Work out the finished part from the listing and answer in its coordinate system (mm). Face numbers are marked on the shaded views. A direction names the side the tool comes from. Give positions to 0.01 mm unless a question says otherwise; leave off trailing zeros. Order: outer loops, then holes, each group sorted by start corner. A loop starts at its lowest first (then second) coordinate and runs counter-clockwise, first axis right, second up. Notation, with made-up numbers: (32.5, -13.5) - (78.5, -13.5) arc R31 cw to (78.5, 21.5) - close; hole circle Ø7 at (-20, 68.25). An arc over 180 degrees is marked (long way). Put each result on its own line as item: value.
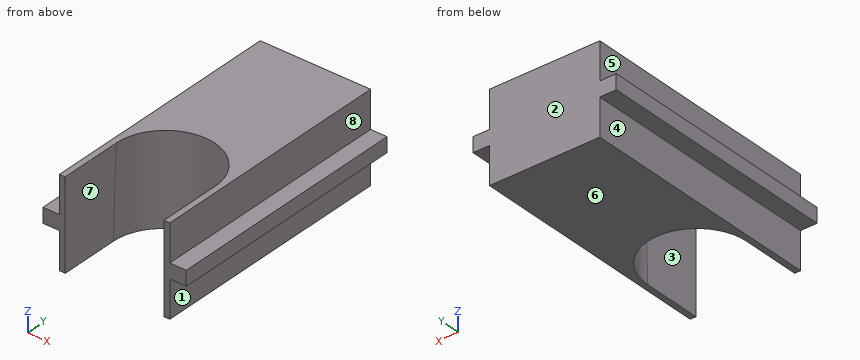
Autodesk Inventor part; units mm, degrees
ref_plane "YZ Plane" through (0, 0, 0) normal (1, 0, 0) x (0, 1, 0)
ref_plane "XZ Plane" through (0, 0, 0) normal (0, 1, 0) x (-1, 0, 0)
ref_plane "XY Plane" through (0, 0, 0) normal (0, 0, 1) x (1, 0, 0)
sketch "草圖1" plane through (0, 0, 0) normal (0, 1, 0) x (-1, 0, 0)
  line L0 (-33.5, 27) -> (33.5, 27)
  line L1 (33.5, 27) -> (33.5, -27)
  line L2 (33.5, -27) -> (-33.5, -27)
  line L3 (-33.5, -27) -> (-33.5, 27)
  line L4 (-33.5, 27) -> (33.5, -27) construction
  line L5 (33.5, 27) -> (-33.5, -27) construction
  line L6 (43.5, -4.5) -> (33.5, -4.5)
  line L7 (33.5, -4.5) -> (33.5, 4.5)
  line L8 (33.5, 4.5) -> (43.5, 4.5)
  line L9 (43.5, 4.5) -> (43.5, -4.5)
  line L10 (-33.5, -4.5) -> (-43.5, -4.5)
  line L11 (-43.5, -4.5) -> (-43.5, 4.5)
  line L12 (-43.5, 4.5) -> (-33.5, 4.5)
  line L13 (-33.5, 4.5) -> (-33.5, -4.5)
  point P0 (0, 0)
  point P1 (33.5, 0)
  point P2 (-33.5, 0)
  point P3 (-33.5, 4.5)
  point P4 (-33.5, -4.5)
  dimension "d0" = 67
  dimension "d1" = 54
  dimension "d2" = 9
  dimension "d3" = 10
extrude "擠出1" add sketch "草圖1" along normal blind 200
sketch "草圖2" plane through (-33.5, 0, 27) normal (0, 0, 1) x (1, 0, 0)
  circle A0 centre (33.5, 78) radius 30
  line L0 (0, 0) -> (67, 0)
  line L1 (3.5, 78) -> (63.5, 78)
  line L2 (63.5, 78) -> (63.5, -10.8713)
  line L3 (63.5, -10.8713) -> (3.5, -10.8713)
  line L4 (3.5, -10.8713) -> (3.5, 78)
  point P0 (33.5, 0)
  point P1 (33.5, 0)
  point P2 (63.5, 78)
  dimension "d6" = 78
  dimension "d7" = 60
extrude "擠出2" cut sketch "草圖2" against normal through all
sketch "草圖3" plane through (-33.5, 200, 27) normal (0, 0, 1) x (1, 0, 0)
  line L0 (-51.5496, -150) -> (118.5496, -150)
  line L1 (118.5496, -150) -> (118.5496, -200)
  line L2 (118.5496, -200) -> (-51.5496, -200)
  line L3 (-51.5496, -200) -> (-51.5496, -150)
  point P0 (33.5, -200)
  point P1 (33.5, -200)
  dimension "d10" = 50
extrude "擠出3" cut sketch "草圖3" against normal through all
sketch "草圖4" plane through (33.5, 200, -27) normal (0, 0, -1) x (-1, 0, 0)
  arc A0 (63.5, -122) -> (3.5, -122) centre (33.5, -122) ccw construction
  circle A1 centre (33.5, -114) radius 30
  line L0 (63.5, -150) -> (3.5, -150)
  line L1 (3.5, -150) -> (3.5, -114)
  line L2 (3.5, -114) -> (63.5, -114)
  line L3 (63.5, -114) -> (63.5, -150)
  point P0 (33.5, -200)
  point P1 (63.5, -150)
  dimension "d13" = 8
  dimension "d14" = 60
sketch "草圖5" plane through (-33.5, 200, 27) normal (0, 0, 1) x (1, 0, 0)
  arc A0 (63.5, -122) -> (3.5, -122) centre (33.5, -122) ccw construction
  circle A1 centre (33.5, -112) radius 30
  line L0 (63.5, -150) -> (3.5, -150)
  line L1 (3.5, -150) -> (3.5, -112)
  line L2 (3.5, -112) -> (63.5, -112)
  line L3 (63.5, -112) -> (63.5, -150)
  point P0 (33.5, -200)
  point P1 (63.5, -150)
  dimension "d15" = 10
  dimension "d16" = 60
loft "斷面混成1" cut profiles "草圖4", "草圖5"
properties part number "Slider-3"
(1) Given pin 1 (3 mm diameter, centred on x = 22.5, z = -14.5, fed in from -Y); pin 2 (7 mm diameter, centred on y = 106, z = -17, fed in from -X); pin 3 (25 mm diameter, centred on y = 109.5, z = -18, fed in from +X); pin 4 (25 mm diameter, centred on y = 120, z = 11.5, fed in from -X), each flat-ended and moving along its own axis, determine where each tip first touches the part or whether it passes through.
Geometry check:
pin 1: stops at y = 104.46
pin 2: stops at x = -33.5
pin 3: stops at x = 33.5
pin 4: stops at x = -43.5
(2) Straight lines are drawn through the part: line 1 (X direction, y = 70.5, z = 12); line 2 (X direction, y = 96, z = -7); line 3 (Z direction, x = -39, y = 116.5). For each, find the intervals that lie inside material, in ascending order.
Geometry check:
line 1: x = -33.5 to -30, 30 to 33.5
line 2: x = -33.5 to -28.54, 28.54 to 33.5
line 3: z = -4.5 to 4.5
(3) Section A-A, the plane y = 168.5 is taken. Write down the section's boundary in (x, z).
Geometry check:
outline: (-43.5, -4.5) - (-33.5, -4.5) - (-33.5, -27) - (33.5, -27) - (33.5, -4.5) - (43.5, -4.5) - (43.5, 4.5) - (33.5, 4.5) - (33.5, 27) - (-33.5, 27) - (-33.5, 4.5) - (-43.5, 4.5) - close
(4) A tool of negligible diameter and unlimited length cuts with its end or side. For the marked faces 1, 2, 3, 4 and 5, from which of +Z, -Z, +X, -X, +Y, -Y can it reach the whole face along a straight path? Write none if from no direction.
Geometry check:
face 1: -Z, +X, +Y, -Y
face 2: +Z, -Z, +X, -X, +Y
face 3: +Z, -Z, -Y
face 4: -Z, -X, +Y, -Y
face 5: +Z, -X, +Y, -Y
(5) Determine the mould class of the marked faces 6, 7 and 8 for opening direction X: pulls with the +X half, pulls with the -X half, needs draft (parallel to the pull), parting line crosses it, or undercut.
Geometry check:
face 6: needs draft
face 7: undercut
face 8: pulls with the +X half
